The model under review builds one solid part; all positions refer to its coordinate system, in mm. Face numbers are marked on the shaded views. A direction names the side the tool comes from. Give positions to 0.01 mm unless a question says otherwise; leave off trailing zeros. Order: outer loops, then holes, each group sorted by start corner. A loop starts at its lowest first (then second) coordinate and runs counter-clockwise, first axis right, second up. Notation, with made-up numbers: M -39.75,68 L -3.75,68 A24 ccw -3.75,102 Z; hole C -8.5,-32 d2. An arc over 180 degrees is marked long. One line per question, with ' | ' between items. Start each with the question number.
1. Wall thickness on L1, parallel to X at y = -9, z = 11; L2, parallel to Y at x = 46, z = 0.55; L3, parallel to Z at x = 21, y = 13: over which ranges is each line inside the solid? List them lowest first.
2. We need section D-D on y = -22. Write out the cut boundary in (x, z).
3. For the marked faces 1 and 2, list the 3-axis set-ups (+Z, -Z, +X, -X, +Y, -Y) from which the entire face can be reached by the end or side of a thin tool; tool diameter is ignored.
4. Insertion check: P1, Ø4, axis at x = -7, z = 18, coming from the +Y side; P2, Ø9, axis at x = -8.5, y = 17.5, coming from the +Z side; P3, Ø1.5, axis at x = -4, y = -5, coming from the +Z side. Each pin has a flat end and moves straight along its axis. Give the tip position at first contact, or say it passes through.
5. The part is to be moulded in two halves that separate along X. For the marked faces 3, 4 and 5, say which applies: +X half, -X half, draft (parallel to the pull), parting line (faces both ways), or undercut.
6. We need section A-A on x = 23. Write out the cut boundary in (y, z).
7. We need section C-C on x = 46. Write out the cut boundary in (y, z), then the cut area to 3 significant figures.
8. We need section B-B on z = 18. Count the separate pieces of the cut face and the enclosed holes in it, then the cut area to 3 significant figures.
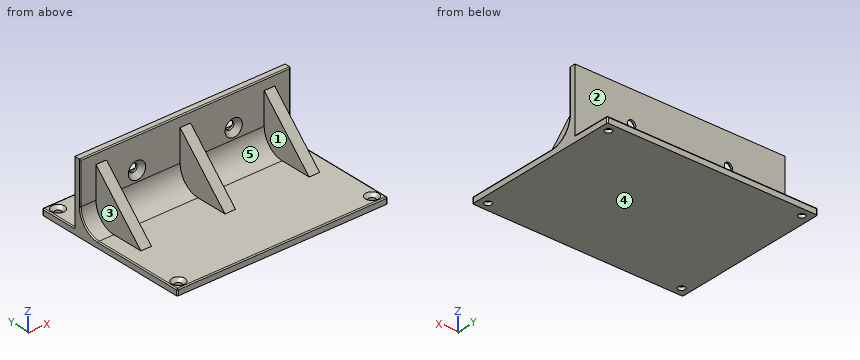
```python
from build123d import *

# Parameters (mm, degrees)
SZKIC1_W                                             = 100
SZKIC1_H                                             = 75
DODANIE_WYCI_GNI_CIE1_DEPTH                          = 3
SZKIC2_W                                             = 30
SZKIC2_H                                             = 3
DODANIE_WYCI_GNI_CIE2_DEPTH                          = 100
EBRO6_REACH                                          = 98.1
SZKIC3_WALL_W                                        = 229.555755292
SZKIC3_WALL_H                                        = 5
SZYK_LINIOWY1_COUNT                                  = 2
SZYK_LINIOWY1_PITCH                                  = 40
SZYK_LINIOWY2_COUNT                                  = 2
SZYK_LINIOWY2_PITCH                                  = 40
SZKIC4_R                                             = 1.6
WYTNIJ_WYCI_GNI_CIE1_DEPTH                           = 77.732214276
SFAZOWANIE1_SIZE                                     = 1.5
POG_BIENIE_STO_KOWE_POD_M3_5_WKR_T_DO_CZ_D           = 3.9
POG_BIENIE_STO_KOWE_POD_M3_5_WKR_T_DO_CZ_CSINK_D     = 8.2
POG_BIENIE_STO_KOWE_POD_M3_5_WKR_T_DO_CZ_CSINK_ANGLE = 90
ZAOKR_GLENIE1_R                                      = 10
ZAOKR_GLENIE2_R                                      = 0.5


with BuildPart() as part:
    # Szkic1 → Dodanie-wyciągnięcie1 (new body)
    with BuildSketch(Plane.XY):
        with Locations((0, -12.378178673)):
            Rectangle(SZKIC1_W, SZKIC1_H)
    extrude(amount=DODANIE_WYCI_GNI_CIE1_DEPTH)

    # Szkic2 → Dodanie-wyciągnięcie2 (add)
    with BuildSketch(Plane.ZY.offset(50)):
        with Locations((18, 5.621821327)):
            Rectangle(SZKIC2_W, SZKIC2_H)
    extrude(amount=-DODANIE_WYCI_GNI_CIE2_DEPTH)

    # Szkic3 wall → Żebro6 (add, up to next)
    with BuildSketch(Plane(origin=(0, -8.378178673, 15.5), x_dir=(0, -0.707106781187, -0.707106781187), z_dir=(0, 0.707106781187, -0.707106781187)), mode=Mode.PRIVATE) as ebro6_sk1:
        Rectangle(SZKIC3_WALL_W, SZKIC3_WALL_H)
    ebro6_tool1 = extrude(ebro6_sk1.sketch, amount=EBRO6_REACH, mode=Mode.PRIVATE) - part.part
    ebro6 = ebro6_tool1.solids().sort_by_distance((0, -8.378178673, 15.5))[0]
    add(ebro6)

    # Szyk liniowy1: Żebro6 ×2
    with Locations(*[(-i * SZYK_LINIOWY1_PITCH, 0, 0) for i in range(1, SZYK_LINIOWY1_COUNT)]):
        add(ebro6)

    # Szyk liniowy2: Żebro6 ×2
    with Locations(*[(i * SZYK_LINIOWY2_PITCH, 0, 0) for i in range(1, SZYK_LINIOWY2_COUNT)]):
        add(ebro6)

    # Szkic4 → Wytnij-wyciągnięcie1 (cut, through all)
    with BuildSketch(Plane.XY.offset(3)):
        with Locations((46, -45.878178673)):
            Circle(SZKIC4_R)
        with Locations((-46, -45.878178673)):
            Circle(SZKIC4_R)
        with Locations((46, 21.121821327)):
            Circle(SZKIC4_R)
        with Locations((-46, 21.121821327)):
            Circle(SZKIC4_R)
    extrude(amount=-WYTNIJ_WYCI_GNI_CIE1_DEPTH, mode=Mode.SUBTRACT)

    # Sfazowanie1
    sfazowanie1_edges = [part.edges().sort_by_distance(p)[0] for p in [
        (-47.6, -45.878178673, 3),
        (44.4, 21.121821327, 3),
        (-47.6, 21.121821327, 3),
        (44.4, -45.878178673, 3),
    ]]
    chamfer(sfazowanie1_edges, length=SFAZOWANIE1_SIZE)

    # Pogłębienie stożkowe pod M3.5 wkręt do części metalowych z łbem soczewkowym1 (through all)
    with Locations(Plane(origin=(0, 4.121821327, 0), x_dir=(-1, 0, 0), z_dir=(0, -1, 0))):
        with Locations((-23, -18), (23, -18)):
            CounterSinkHole(POG_BIENIE_STO_KOWE_POD_M3_5_WKR_T_DO_CZ_D / 2, POG_BIENIE_STO_KOWE_POD_M3_5_WKR_T_DO_CZ_CSINK_D / 2, counter_sink_angle=POG_BIENIE_STO_KOWE_POD_M3_5_WKR_T_DO_CZ_CSINK_ANGLE)

    # Zaokrąglenie1
    zaokr_glenie1_edges = [part.edges().sort_by_distance(p)[0] for p in [
        (46.25, 4.121821327, 3),
        (-20, 4.121821327, 3),
        (-46.25, 4.121821327, 3),
        (20, 4.121821327, 3),
    ]]
    fillet(zaokr_glenie1_edges, radius=ZAOKR_GLENIE1_R)

    # Zaokrąglenie2
    zaokr_glenie2_edges = [part.edges().sort_by_distance(p)[0] for p in [
        (-50, 16.121821327, 3),
        (50, 16.121821327, 3),
        (-50, -27.878178673, 3),
        (-50, 4.121821327, 23),
        (50, 1.192889139, 5.928932188),
        (-50, 1.192889139, 5.928932188),
        (0, 4.121821327, 33),
        (0, -49.878178673, 3),
        (50, 4.121821327, 23),
        (50, -27.878178673, 3),
        (50, -49.878178673, 1.5),
        (-50, -49.878178673, 1.5),
        (-50, 25.121821327, 1.5),
        (50, 25.121821327, 1.5),
        (0, 25.121821327, 3),
    ]]
    fillet(zaokr_glenie2_edges, radius=ZAOKR_GLENIE2_R)


solid = part.part
```
Entries:
1) L1: x = -42.5 to -37.5, -2.5 to 2.5, 37.5 to 42.5 | L2: y = -49.88 to -47.48, -44.28 to 19.52, 22.72 to 25.12 | L3: z = 0 to 3
2) outline: M -50,0 L 50,0 L 50,2.5 A0.5 ccw 49.5,3 L -49.5,3 A0.5 ccw -50,2.5 Z
3) face 1: +Z, -Y | face 2: +Z, +X, -X, +Y
4) P1: stops at y = 7.12 | P2: stops at z = 3 | P3: stops at z = 3.13
5) face 3: -X half | face 4: draft | face 5: undercut
6) outline: M -49.88,0 L 25.12,0 L 25.12,2.5 A0.5 ccw 24.62,3 L 7.12,3 L 7.12,16.05 L 6.27,16.05 L 4.12,13.9 L 4.12,13 A10 cw -5.88,3 L -49.38,3 A0.5 ccw -49.88,2.5 Z; M 4.12,22.1 L 6.27,19.95 L 7.12,19.95 L 7.12,33 L 4.62,33 A0.5 ccw 4.12,32.5 Z
7) outline: M -49.88,0 L -47.48,0 L -47.48,1.5 L -48.98,3 L -49.38,3 A0.5 ccw -49.88,2.5 Z; M -44.28,0 L 19.52,0 L 19.52,1.5 L 18.02,3 L 7.12,3 L 7.12,33 L 4.62,33 A0.5 ccw 4.12,32.5 L 4.12,13 A10 cw -5.88,3 L -42.78,3 L -44.28,1.5 Z; M 22.72,0 L 25.12,0 L 25.12,2.5 A0.5 ccw 24.62,3 L 24.22,3 L 22.72,1.5 Z | area: 313 mm^2
8) separate pieces: 3 | enclosed holes: 0 | area: 417 mm^2
